Build history of the part. All positions in model axes, mm. Give positions to 0.01 mm unless a question says otherwise; leave off trailing zeros. Order: outer loops, then holes, each group sorted by start corner. A loop starts at its lowest first (then second) coordinate and runs counter-clockwise, first axis right, second up. Notation, with made-up numbers: M 65.25,38.25 L 116.25,38.25 A13 ccw 116.25,53.25 Z; hole C 9,-3 d7. An arc over 180 degrees is marked long. One line per item, written item: value.
from build123d import *

# Parameters (mm, degrees)
SKETCH1_W           = 150
SKETCH1_H           = 225
BOSS_EXTRUDE1_DEPTH = 5
SKETCH10_W          = 25
SKETCH10_H          = 5
CUT_EXTRUDE5_DEPTH  = 5
SKETCH11_W          = 15
SKETCH11_H          = 5
CUT_EXTRUDE6_DEPTH  = 5
SKETCH12_W          = 5
SKETCH12_H          = 15
CUT_EXTRUDE7_DEPTH  = 5
SKETCH13_R          = 2
CUT_EXTRUDE8_DEPTH  = 5
SKETCH14_W          = 20
SKETCH14_H          = 20
CUT_EXTRUDE9_DEPTH  = 5
SKETCH15_W          = 5
SKETCH15_H          = 25
CUT_EXTRUDE10_DEPTH = 5


with BuildPart() as part:
    # Sketch1 → Boss-Extrude1 (new body)
    with BuildSketch(Plane(origin=(0, 0, 0), x_dir=(1, 0, 0), z_dir=(0, 1, 0))):
        Rectangle(SKETCH1_W, SKETCH1_H)
    extrude(amount=BOSS_EXTRUDE1_DEPTH)

    # Sketch10 → Cut-Extrude5 (cut)
    with BuildSketch(Plane(origin=(0, 5, 0), x_dir=(1, 0, 0), z_dir=(0, 1, 0))):
        with Locations((-55.5, -103)):
            Rectangle(SKETCH10_W, SKETCH10_H)
        with Locations((-55.5, 103)):
            Rectangle(SKETCH10_W, SKETCH10_H)
        with Locations((55.5, -103)):
            Rectangle(SKETCH10_W, SKETCH10_H)
        with Locations((55.5, 103)):
            Rectangle(SKETCH10_W, SKETCH10_H)
    extrude(amount=-CUT_EXTRUDE5_DEPTH, mode=Mode.SUBTRACT)

    # Sketch11 → Cut-Extrude6 (cut)
    with BuildSketch(Plane(origin=(0, 5, 0), x_dir=(1, 0, 0), z_dir=(0, 1, 0))):
        with Locations((-60.5, 90.5)):
            Rectangle(SKETCH11_W, SKETCH11_H)
        with Locations((60.5, 90.5)):
            Rectangle(SKETCH11_W, SKETCH11_H)
        with Locations((-60.5, 60.5)):
            Rectangle(SKETCH11_W, SKETCH11_H)
        with Locations((60.5, 60.5)):
            Rectangle(SKETCH11_W, SKETCH11_H)
    extrude(amount=-CUT_EXTRUDE6_DEPTH, mode=Mode.SUBTRACT)

    # Sketch12 → Cut-Extrude7 (cut)
    with BuildSketch(Plane(origin=(0, 5, 0), x_dir=(1, 0, 0), z_dir=(0, 1, 0))):
        with Locations((-65.5, -30)):
            Rectangle(SKETCH12_W, SKETCH12_H)
        with Locations((65.5, -30)):
            Rectangle(SKETCH12_W, SKETCH12_H)
    extrude(amount=-CUT_EXTRUDE7_DEPTH, mode=Mode.SUBTRACT)

    # Sketch13 → Cut-Extrude8 (cut)
    with BuildSketch(Plane(origin=(0, 5, 0), x_dir=(1, 0, 0), z_dir=(0, 1, 0))):
        with Locations(Location((-65.5, -62.5, 0), (0, 0, 270))):
            Circle(SKETCH13_R)
        with Locations(Location((-65.5, -91.5, 0), (0, 0, 270))):
            Circle(SKETCH13_R)
        with Locations(Location((65.5, -91.5, 0), (0, 0, 270))):
            Circle(SKETCH13_R)
        with Locations(Location((65.5, -62.5, 0), (0, 0, 270))):
            Circle(SKETCH13_R)
    extrude(amount=-CUT_EXTRUDE8_DEPTH, mode=Mode.SUBTRACT)

    # Sketch14 → Cut-Extrude9 (cut)
    with BuildSketch(Plane(origin=(0, 5, 0), x_dir=(1, 0, 0), z_dir=(0, 1, 0))):
        with Locations((20, 72.5)):
            Rectangle(SKETCH14_W, SKETCH14_H)
        with Locations((-20, 72.5)):
            Rectangle(SKETCH14_W, SKETCH14_H)
    extrude(amount=-CUT_EXTRUDE9_DEPTH, mode=Mode.SUBTRACT)

    # Sketch15 → Cut-Extrude10 (cut)
    with BuildSketch(Plane(origin=(0, 5, 0), x_dir=(1, 0, 0), z_dir=(0, 1, 0))):
        with Locations((0, 88)):
            Rectangle(SKETCH15_W, SKETCH15_H)
    extrude(amount=-CUT_EXTRUDE10_DEPTH, mode=Mode.SUBTRACT)


solid = part.part
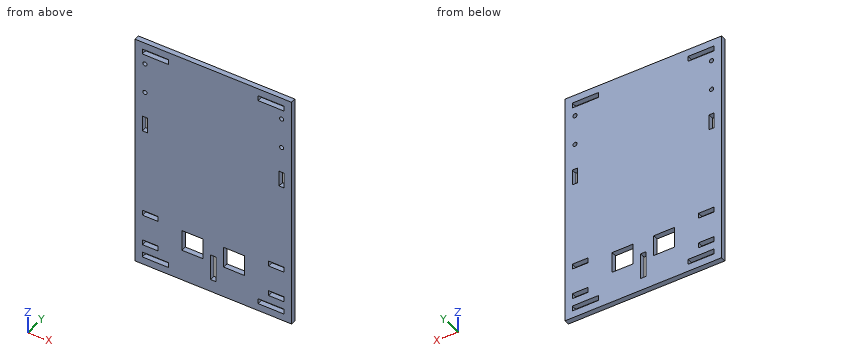
1) Saw through at C-C, the plane z = 25. Write the cut outline in (x, y), then the cut area to 3 significant figures.
Check values:
outline: M -75,0 L -68,0 L -68,5 L -75,5 Z; M -63,0 L 63,0 L 63,5 L -63,5 Z; M 68,0 L 75,0 L 75,5 L 68,5 Z
area: 700 mm^2
2) Saw through at D-D, the plane y = 1.8. Give the number of separate pieces and of enclosed holes in the cut face, then the cut area to 3 significant figures.
Check values:
separate pieces: 1
enclosed holes: 17
area: 31,800 mm^2
3) Drill centre lines: probe 1 along X at (y, z) = (1.75, 91.5); probe 2 along Z at (x, y) = (59, 2.9); probe 3 along Z at (x, y) = (-26.5, 2.2). Where is each one in solid material? Low to high. Write a range as from..to.
Check values:
probe 1: -75..-67.5, -63.5..63.5, 67.5..75
probe 2: -112.5..-105.5, -100.5..-93, -88..-63, -58..100.5, 105.5..112.5
probe 3: -112.5..-82.5, -62.5..112.5
4) Saw through at B-B, the plane x = -20. Write the cut outline in (y, z).
Check values:
outline: M 0,-112.5 L 5,-112.5 L 5,-82.5 L 0,-82.5 Z; M 0,-62.5 L 5,-62.5 L 5,112.5 L 0,112.5 Z
5) Saw through at A-A, the plane z = -79. Write the cut outline in (x, y).
Check values:
outline: M -75,0 L -30,0 L -30,5 L -75,5 Z; M -10,0 L -2.5,0 L -2.5,5 L -10,5 Z; M 2.5,0 L 10,0 L 10,5 L 2.5,5 Z; M 30,0 L 75,0 L 75,5 L 30,5 Z
6) Pin check, flat tip, straight feed: pin 1 (6 mm diameter, centred on x = 22, z = -62, fed in from -Y). Stop position of the tip, or through.
Check values:
pin 1: y = 0
